Here's how the part is built. I have some questions about the finished solid (model axes, mm). Give positions to 0.01 mm unless a question says otherwise; leave off trailing zeros. Loops run counter-clockwise (first coordinate to the right, second up) from the corner with the lowest first, then second, coordinate; pieces in that order, holes last. Notation, with made-up numbers: (40.25, -7) - (59.25, -7) arc R20 ccw to (59.25, 7) - close; hole circle Ø4 at (55, -8). An arc over 180 degrees is marked (long way). Use one line per item in the form item = value.
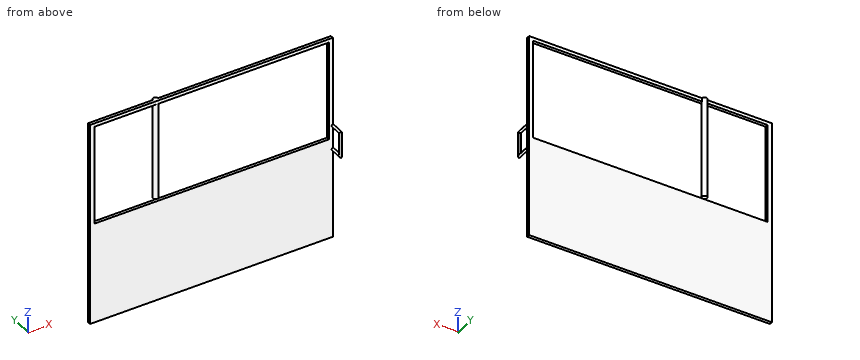
from build123d import *

# Parameters (mm, degrees)
F1_DEPTH = 25
F5_W     = 1931.8042993546
F5_H     = 827.8105258942
F6_DEPTH = 25


with BuildPart() as f1:
    # F0 (on Front) → F1 (new body)
    with BuildSketch(Plane.XZ):
        Polygon((-1000, 0), (0, 0), (1000, 0), (1000, 1700), (0, 1700), (-1000, 1700), align=None)
    extrude(amount=F1_DEPTH)

    # F4: sweep along a path in F2
    with BuildLine(Plane.YZ.offset(1000)) as f4_path:
        Line((-25, 950), (-125, 950))
        Line((-125, 950), (-125, 750))
        Line((-125, 750), (-25, 750))
    # F3 (on face) → F4 (sweep)
    with BuildSketch(Plane.XZ.offset(25)):
        with BuildLine():
            ThreePointArc((1000, 940.1793980598), (1007.0710678119, 943.108330248), (1010, 950.1793980598))
            ThreePointArc((1010, 950.1793980598), (1007.0710678119, 957.2504658717), (1000, 960.1793980598))
            Line((1000, 960.1793980598), (1000, 940.1793980598))
        make_face()
        with BuildLine():
            Line((1000, 940.1793980598), (1000, 960.1793980598))
            ThreePointArc((1000, 960.1793980598), (990, 950.1793980598), (1000, 940.1793980598))
        make_face()
    sweep(path=f4_path.line, transition=Transition.RIGHT)

    # F5 (on face) → F6 (cut)
    with BuildSketch(Plane.XZ.offset(25)):
        with Locations((2.4275183678, 1257.6580047607)):
            Rectangle(F5_W, F5_H)
    extrude(amount=-F6_DEPTH, mode=Mode.SUBTRACT)

    # F9: sweep along a path in F7
    with BuildLine(Plane.XZ) as f9_path:
        Line((0, 847.6967215538), (0, 1689.0659332275))
    # F8 (on face) → F9 (sweep)
    with BuildSketch(Plane.XY.offset(1700)):
        with BuildLine():
            ThreePointArc((-464.7935223579, 0), (-444.7935223579, -20), (-424.7935223579, 0))
            Line((-424.7935223579, 0), (-464.7935223579, 0))
        make_face()
        with BuildLine():
            Line((-464.7935223579, 0), (-424.7935223579, 0))
            ThreePointArc((-424.7935223579, 0), (-444.7935223579, 20), (-464.7935223579, 0))
        make_face()
    sweep(path=f9_path.line)


solid = f1.part
(1) If we section it at A-A (x = 756): List the corners of the cut face in (y, z) for me, plus the area to 3 significant figures.
Geometry says:
outline = (-25, 0) - (0, 0) - (0, 843.75) - (-25, 843.75) - close; (-25, 1671.56) - (0, 1671.56) - (0, 1700) - (-25, 1700) - close
area = 21,800 mm²
(2) For P1, Ø12.5, axis at y = -13.5, z = 804.5, coming from the +X side; P2, Ø20, axis at x = 455, y = -15.5, coming from the -Z side; P3, Ø8, axis at x = 1005.5, z = 748.5, coming from the +Y side; P4, Ø8, axis at x = 321.5, z = 205.5, coming from the +Y side, each with a flat end and sliding along its axis, tell me the tip position at first contact or that it passes through.
Geometry says:
P1 = 1000
P2 = 0
P3 = -25
P4 = 0
(3) If we section it at C-C (y = -74): List the corners of the cut face in (x, z) for me.
Geometry says:
outline = circle Ø20 at (1000, 749.82); circle Ø20 at (1000, 950.18)
(4) If I drill on probe 1 along X at (y, z) = (-7, 1021); probe 2 along Y at (x, z) = (-21, 92.5); probe 3 along X at (y, z) = (-21, 1014), over which ranges is the centre line in solid material (lowest first)?
Geometry says:
probe_1 = -1000 to -963.47, -463.53 to -426.06, 968.33 to 1000
probe_2 = -25 to 0
probe_3 = -1000 to -963.47, 968.33 to 1000
(5) If we section it at B-B (z = 1597): List the corners of the cut face in (x, y) for me, plus the area to 3 significant figures.
Geometry says:
outline = (-1000, -25) - (-963.47, -25) - (-963.47, 0) - (-1000, 0) - close; circle Ø40 at (-444.79, 0); (968.33, -25) - (1000, -25) - (1000, 0) - (968.33, 0) - close
area = 2,960 mm²
(6) If we section it at D-D (z = 637): List the corners of the cut face in (x, y) for me, plus the area to 3 significant figures.
Geometry says:
outline = (-1000, -25) - (1000, -25) - (1000, 0) - (-1000, 0) - close
area = 50,000 mm²
